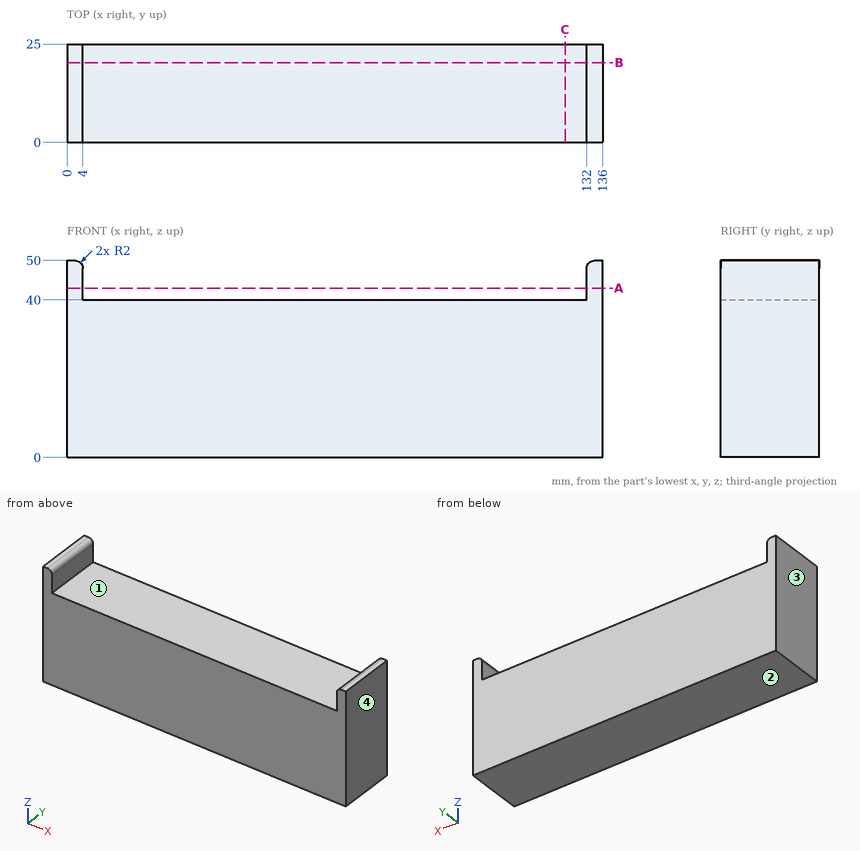
Source: three-view drawing plus pictorial views. Frame: mm from the lowest corner of the part. Round coordinates to 2 decimals unless told otherwise and drop trailing zeros. Order: outer loops, then holes, each group sorted by start corner. A loop starts at its lowest first (then second) coordinate and runs counter-clockwise, first axis right, second up. Notation, with made-up numbers: (-6.75, 21) - (21.25, 21) arc R16 ccw to (21.25, 27) - close; hole circle Ø1 at (-23, -24.5). An arc over 180 degrees is marked (long way). Answer in a Markdown table with one row per item.
Item 1: Line query: line 1 (X direction, y = 22.75, z = 46); line 2 (Z direction, x = 130, y = 2). Output: solid intervals per line, ascending.
Model answer:
| item | result |
|---|---|
| line 1 | x = 0 to 4, 132 to 136 |
| line 2 | z = 0 to 40 |
Item 2: Section query B-B (y = 20.25). Return the cut outline in (x, z).
Model answer:
| item | result |
|---|---|
| outline | (0, 0) - (136, 0) - (136, 50) - (134, 50) arc R2 ccw to (132, 48) - (132, 40) - (4, 40) - (4, 48) arc R2 ccw to (2, 50) - (0, 50) - close |
Item 3: Section query C-C (x = 126.5). Return the cut outline in (y, z).
Model answer:
| item | result |
|---|---|
| outline | (0, 0) - (25, 0) - (25, 40) - (0, 40) - close |
Item 4: Mould query, pull axis X, two halves, no side actions, for the marked faces 1, 2, 3 and 4. Classes: released by +X, released by -X, zero draft, split by the parting line, or undercut.
Model answer:
| item | result |
|---|---|
| face 1 | undercut |
| face 2 | zero draft |
| face 3 | released by -X |
| face 4 | released by +X |
Item 5: Section query A-A (z = 43). Return the cut outline in (x, y), then the cut area to 3 significant figures.
Model answer:
| item | result |
|---|---|
| outline | (0, 0) - (4, 0) - (4, 25) - (0, 25) - close; (132, 0) - (136, 0) - (136, 25) - (132, 25) - close |
| area | 200 mm² |
